Check sheet for the drawn part. Datum: minimum x, y, z corner. Units: mm. Round coordinates to 2 decimals unless told otherwise and drop trailing zeros. Write each loop counter-clockwise with the first axis right and the second up, starting at its lowest first coordinate (ties: lowest second). Pieces come first, ordered by that corner, then holes.
Item 1: Go/stop test with a flat-tipped pin: pin 1 Ø2 at (x, y) = (5, 16) entering from -Z. Record where the tip stops, or that it passes through.
Item 2: Cross-section at A-A on x = 5. Enter the section's corners in (y, z).
Item 3: Material ranges on line 1 (Y direction, x = 5, z = 2.1); line 2 (X direction, y = 16, z = 1.55); line 3 (Y direction, x = 5.5, z = 0.45), recorded low to high.
Item 4: Cross-section at B-B on y = 16. Enter the section's corners in (x, z).
Item 5: Cross-section at C-C on z = 2.2. Enter the section's corners in (x, y), plus the area to 3 significant figures.
Item 6: Release check for a two-part mould opening along X. For the marked faces 1, 2, 3 and 4 record: +X half, -X half, draft (parallel to the pull), parting line (faces both ways), or undercut.
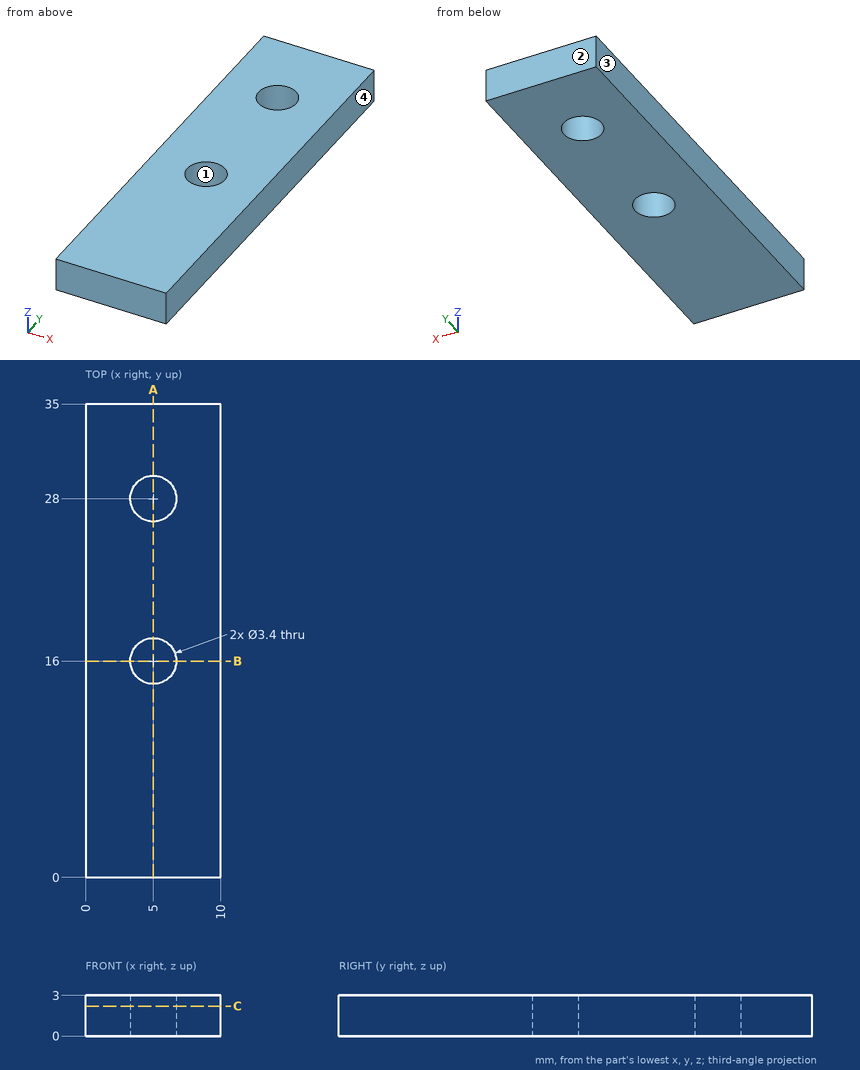
Response values:
1. pin 1: passes through
2. outline: (0, 0) - (14.3, 0) - (14.3, 3) - (0, 3) - close; (17.7, 0) - (26.3, 0) - (26.3, 3) - (17.7, 3) - close; (29.7, 0) - (35, 0) - (35, 3) - (29.7, 3) - close
3. line 1: y = 0 to 14.3, 17.7 to 26.3, 29.7 to 35
3. line 2: x = 0 to 3.3, 6.7 to 10
3. line 3: y = 0 to 14.38, 17.62 to 26.38, 29.62 to 35
4. outline: (0, 0) - (3.3, 0) - (3.3, 3) - (0, 3) - close; (6.7, 0) - (10, 0) - (10, 3) - (6.7, 3) - close
5. outline: (0, 0) - (10, 0) - (10, 35) - (0, 35) - close; hole circle Ø3.4 at (5, 16); hole circle Ø3.4 at (5, 28)
5. area: 332 mm2
6. face 1: undercut
6. face 2: draft
6. face 3: -X half
6. face 4: +X half
